Geometry: final body of the model. Coordinates: model frame, mm. A direction names the side the tool comes from. Give positions to 0.01 mm unless a question says otherwise; leave off trailing zeros. Write each loop counter-clockwise with the first axis right and the second up, starting at its lowest first coordinate (ties: lowest second). Pieces come first, ordered by that corner, then holes. Notation, with made-up numbers: M -22,41 L 22,41 A20 cw 22,53 Z; hole C -9.5,-17.75 d1. An arc over 180 degrees is marked long. Use one line per item in the form item = value. Start each with the question number.
Item 1: Section query B-B on y = -8.75. Return loops of the section in (x, z), then the cut area to 3 significant figures.
Item 2: Material intervals for line 1 along X through (y, z) = (1.7, 4.06); line 2 along Z through (x, y) = (45, -9.5); line 3 along Y through (x, z) = (18, 4), sorted ascending. Write a range as from..to.
Item 3: Section query D-D on y = -4.25. Return loops of the section in (x, z).
Item 4: Access query for faces 1 (the flat face through (23, -5, 1.168)), 2 (the flat face through (12, -2.832, 1)), 3 (the flat face through (45.53, -8, 1)). Directions: +Z, -Z, +X, -X, +Y, -Y. A direction counts if a zero-diameter tool reaches every point of the face in a straight line with its end or side. Return the directions, or none.
Item 5: Section query A-A on z = 4.06. Return loops of the section in (x, y), then the cut area to 3 significant figures.
Item 6: Pull-direction query (X, two-part tool) for faces 4 (the cylindrical face through (46.131, -3.402, 0.592)), 5 (the cylindrical face through (19.32, -3.433, 0.592)), 6 (the cylindrical face through (0.57, -12.23, 0.59)), 7 (the cylindrical face through (30.907, 0.835, 1.52)); classes: released by +X, released by -X, zero draft, split by the parting line, or undercut.
Item 7: Contact query for flat-ended pins moving along their axis: P1, Ø0.9, axis at y = -6.5, z = 1, coming from the +X side; P2, Ø3, axis at x = 43.19, z = 4.06, coming from the -Y side; P3, Ø4, axis at x = 14, y = -4.5, coming from the +Z side. Output: stop coordinate, or through.
Item 8: Section query C-C on x = 34. Return loops of the section in (y, z).
from build123d import *

# Parameters (mm, degrees)
BASE_FLANGE1_DEPTH        = 1.1684
EDGE_FLANGE1_DEPTH        = 60.96
TAP_DRILL_FOR_6_32_TAP1_D = 2.7051
FILLET1_R                 = 2


# Sheet-metal steps are written as plain solids
with BuildPart() as part:
    # Sketch1 → Base-Flange1 (new body)
    with BuildSketch(Plane(origin=(0, 0, 0), x_dir=(1, 0, 0), z_dir=(0, 0, -1))):
        Polygon((0, 0), (60.96, 0), (60.96, 2.8316), (45.53, 2.8316), (45.53, 12.8316), (40.21, 12.8316), (40.21, 2.8316), (25.21, 2.8316), (25.21, 12.8316), (19.89, 12.8316), (19.89, 2.8316), (4.89, 2.8316), (4.89, 12.8316), (0, 12.8316), (0, 2.8316), align=None)
    extrude(amount=-BASE_FLANGE1_DEPTH)

    # Edge-Flange1 section (across the edge) → Edge-Flange1 (add)
    with BuildSketch(Plane(origin=(60.96, 1.1684, 1.1684), x_dir=(0, -1, 0), z_dir=(-1, 0, 0))):
        with BuildLine():
            Line((-1.1684, 1.1684), (-1.1684, 7.5052))
            Line((-1.1684, 7.5052), (0, 7.5052))
            Line((0, 7.5052), (0, 1.1684))
            ThreePointArc((0, 1.1684), (0.342216437, 0.342216437), (1.1684, 0))
            Line((1.1684, 0), (1.1684, -1.1684))
            ThreePointArc((1.1684, -1.1684), (-0.483967126, -0.483967126), (-1.1684, 1.1684))
        make_face()
    extrude(amount=EDGE_FLANGE1_DEPTH)

    # Tap Drill for #6-32 Tap1 (through all)
    with Locations(Plane(origin=(0, 2.3368, 0), x_dir=(1, 0, 0), z_dir=(0, 1, 0))):
        with Locations((2.55, -4.06), (22.87, -4.06), (43.19, -4.06)):
            Hole(TAP_DRILL_FOR_6_32_TAP1_D / 2)

    # Fillet1
    fillet1_edges = [part.edges().sort_by_distance(p)[0] for p in [
        (0, -12.8316, 0.5842),
        (4.89, -12.8316, 0.5842),
        (4.89, -2.8316, 0.5842),
        (19.89, -2.8316, 0.5842),
        (19.89, -12.8316, 0.5842),
        (25.21, -12.8316, 0.5842),
        (25.21, -2.8316, 0.5842),
        (40.21, -2.8316, 0.5842),
        (40.21, -12.8316, 0.5842),
        (45.53, -12.8316, 0.5842),
        (45.53, -2.8316, 0.5842),
        (60.96, -2.8316, 0.5842),
        (60.96, 1.7526, 8.6736),
        (0, 1.7526, 8.6736),
    ]]
    fillet(fillet1_edges, radius=FILLET1_R)


solid = part.part
Answer sheet:
q1.outline = M 0,0 L 4.89,0 L 4.89,1.17 L 0,1.17 Z; M 19.89,0 L 25.21,0 L 25.21,1.17 L 19.89,1.17 Z; M 40.21,0 L 45.53,0 L 45.53,1.17 L 40.21,1.17 Z
q1.area = 18.1 mm2
q2.line_1 = 0..1.2, 3.9..21.52, 24.22..41.84, 44.54..60.96
q2.line_2 = 0..1.17
q2.line_3 = 1.17..2.34
q3.outline = M 0,0 L 4.98,0 L 4.98,1.17 L 0,1.17 Z; M 19.8,0 L 25.3,0 L 25.3,1.17 L 19.8,1.17 Z; M 40.12,0 L 45.62,0 L 45.62,1.17 L 40.12,1.17 Z
q4.face_1 = +Z, +X, -X, -Y
q4.face_2 = +Z, -Z, -Y
q4.face_3 = +Z, -Z, +X, -Y
q5.outline = M 0,1.17 L 1.2,1.17 L 1.2,2.34 L 0,2.34 Z; M 3.9,1.17 L 21.52,1.17 L 21.52,2.34 L 3.9,2.34 Z; M 24.22,1.17 L 41.84,1.17 L 41.84,2.34 L 24.22,2.34 Z; M 44.54,1.17 L 60.96,1.17 L 60.96,2.34 L 44.54,2.34 Z
q5.area = 61.7 mm2
q6.face_4 = released by +X
q6.face_5 = undercut
q6.face_6 = released by -X
q6.face_7 = zero draft
q7.P1 = 45.53
q7.P2 = 1.17
q7.P3 = 1.17
q8.outline = M -2.83,0 L 0,0 A2.34 ccw 2.34,2.34 L 2.34,8.67 L 1.17,8.67 L 1.17,2.34 A1.17 cw 0,1.17 L -2.83,1.17 Z
